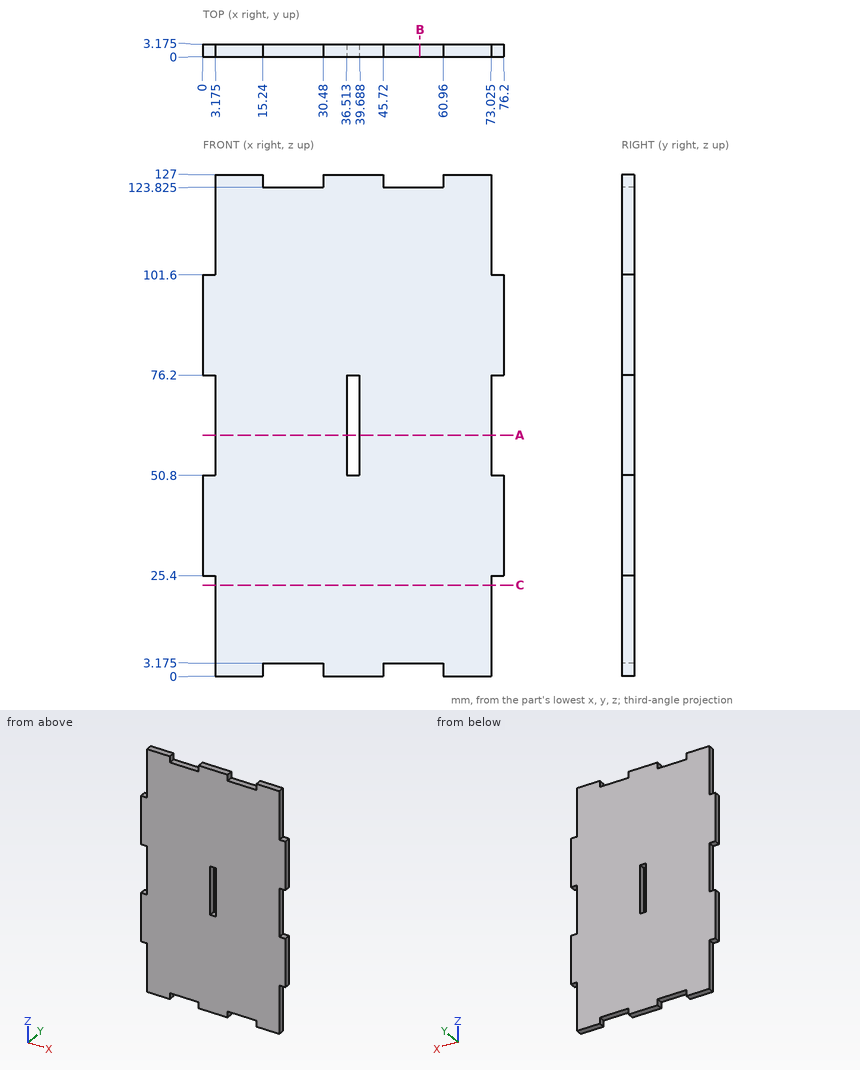
Input: dimensioned drawing with shaded views. Units: mm. Origin: part minimum x, y, z. Coordinates: 2 decimals unless noted, no trailing zeros. Order: outer loops, then holes, each group sorted by start corner. A loop starts at its lowest first (then second) coordinate and runs counter-clockwise, first axis right, second up. Notation, with made-up numbers: (63.25, 18) - (89.25, 18) arc R7 cw to (89.25, 23) - close; hole circle Ø8 at (18.25, 16.5). An arc over 180 degrees is marked (long way). Return JSON: item names as keys, results as strings. Group by question number.
1. Material intervals for line 1 along X through (y, z) = (1.95, 76) (1 decimal); line 2 along X through (y, z) = (2, 103.5) (1 decimal); line 3 along Z through (x, y) = (56.5, 1.7) (1 decimal), sorted ascending. Write a range as [from, to].
2. Cut plane C-C (z = 23). Output: boundary loops of the cut face in (x, y) (1 decimal), plus the area to 3 significant figures.
3. Cut plane B-B (x = 55). Output: boundary loops of the cut face in (y, z) (1 decimal), plus the area to 3 significant figures.
4. Pin query (flat end, axial travel): pin 1 (1.6 mm diameter, centred on x = 74, y = 1, fed in from -Z); pin 2 (1 mm diameter, centred on y = 1, z = 2, fed in from +X) (1 decimal); pin 3 (12 mm diameter, centred on x = 24.5, z = 56, fed in from -Y); pin 4 (1.6 mm diameter, centred on y = 2, z = 67.5, fed in from -X) (1 decimal). Return the tip coordinate at first contact, or that it passes through.
5. Cut plane A-A (z = 61). Output: boundary loops of the cut face in (x, y) (1 decimal), plus the area to 3 significant figures.
Resolved:
{
 "1": {"line 1": "x = [3.2, 36.5], [39.7, 73]", "line 2": "x = [3.2, 73]", "line 3": "z = [3.2, 123.8]"},
 "2": {"outline": "(3.2, 0) - (73, 0) - (73, 3.2) - (3.2, 3.2) - close", "area": "222 mm²"},
 "3": {"outline": "(0, 3.2) - (3.2, 3.2) - (3.2, 123.8) - (0, 123.8) - close", "area": "383 mm²"},
 "4": {"pin 1": "stops at z = 25.4", "pin 2": "stops at x = 73", "pin 3": "stops at y = 0", "pin 4": "stops at x = 3.2"},
 "5": {"outline": "(3.2, 0) - (36.5, 0) - (36.5, 3.2) - (3.2, 3.2) - close; (39.7, 0) - (73, 0) - (73, 3.2) - (39.7, 3.2) - close", "area": "212 mm²"}
}
